Geometry: final body of the model. Coordinates: model frame, mm. A direction names the side the tool comes from. Give positions to 0.01 mm unless a question says otherwise; leave off trailing zeros. Write each loop counter-clockwise with the first axis right and the second up, starting at its lowest first coordinate (ties: lowest second). Pieces come first, ordered by that corner, then holes.
Q1. Cut plane D-D on x = 26. Return the cut outline in (y, z), plus the area to 3 significant figures.
Q2. Line query: L1, parallel to Z at x = 9, y = 2.5; L2, parallel to Y at x = 16, z = -60; L3, parallel to X at y = 0.7, z = -32. Output: solid intervals per line, ascending.
Q3. Cut plane C-C on z = -18.5. Return the cut outline in (x, y).
Q4. Cut plane A-A on x = 4.5. Return the cut outline in (y, z).
Q5. Reachability of faces 1 (the face through (-2, 1, -57)), 2 (the face through (3, 3, -9)), 3 (the face through (10, 3, -5)) from +Z, -Z, +X, -X, +Y, -Y: full face, straight path, thin tool, end or side. Return the list, or none.
Q6. Pin query (flat end, axial travel): pin 1 (1.5 mm diameter, centred on x = 7, y = 3.5, fed in from +Z); pin 2 (0.8 mm diameter, centred on y = 0.5, z = -79.5, fed in from -X); pin 3 (4 mm diameter, centred on x = 1.5, z = -24, fed in from +Y). Return the tip coordinate at first contact, or that it passes through.
Q7. Cut plane B-B on y = 2.15. Return the cut outline in (x, z).
```python
from build123d import *

# Parameters (mm, degrees)
EXTRUDE_1_DEPTH = 1
SKETCH_2_W      = 13
SKETCH_2_H      = 7
EXTRUDE_2_DEPTH = 5
SKETCH_3_W      = 14
SKETCH_3_H      = 13
EXTRUDE_3_DEPTH = 5


with BuildPart() as part:
    # 草圖1 → 填料-伸長1 (new body)
    with BuildSketch(Plane(origin=(0, 0, 0), x_dir=(1, 0, 0), z_dir=(0, 1, 0))):
        Polygon((0, 0), (32, 0), (32, 30), (21, 30), (21, 75), (14.636038969, 81.363961031), (0, 81.363961031), (0, 75.363961031), (11, 75.363961031), (11, 73.363961031), (0, 73.363961031), align=None)
    extrude(amount=EXTRUDE_1_DEPTH)

    # 草圖2 → 填料-伸長2 (add)
    with BuildSketch(Plane(origin=(0, 1, 0), x_dir=(1, 0, 0), z_dir=(0, 1, 0))):
        with Locations((3.5, 5.5)):
            Rectangle(SKETCH_2_W, SKETCH_2_H)
    extrude(amount=EXTRUDE_2_DEPTH)

    # 草圖3 → 填料-伸長3 (add)
    with BuildSketch(Plane(origin=(0, 1, 0), x_dir=(1, 0, 0), z_dir=(0, 1, 0))):
        with Locations((4, 56.863961031)):
            Rectangle(SKETCH_3_W, SKETCH_3_H)
    extrude(amount=EXTRUDE_3_DEPTH)


solid = part.part
```
Data:
1. outline: (0, -30) - (1, -30) - (1, 0) - (0, 0) - close
1. area: 30.0 mm2
2. L1: z = -63.36 to -50.36, -9 to -2
2. L2: y = 0 to 1
2. L3: x = 0 to 21
3. outline: (0, 0) - (32, 0) - (32, 1) - (0, 1) - close
4. outline: (0, -81.36) - (1, -81.36) - (1, -75.36) - (0, -75.36) - close; (0, -73.36) - (1, -73.36) - (1, -63.36) - (6, -63.36) - (6, -50.36) - (1, -50.36) - (1, -9) - (6, -9) - (6, -2) - (1, -2) - (1, 0) - (0, 0) - close
5. face 1: +Z, -Z, -X, -Y
5. face 2: +X, -X, +Y
5. face 3: +Z, +X, +Y
6. pin 1: stops at z = -2
6. pin 2: stops at x = 0
6. pin 3: stops at y = 1
7. outline: (-3, -63.36) - (11, -63.36) - (11, -50.36) - (-3, -50.36) - close; (-3, -9) - (10, -9) - (10, -2) - (-3, -2) - close
